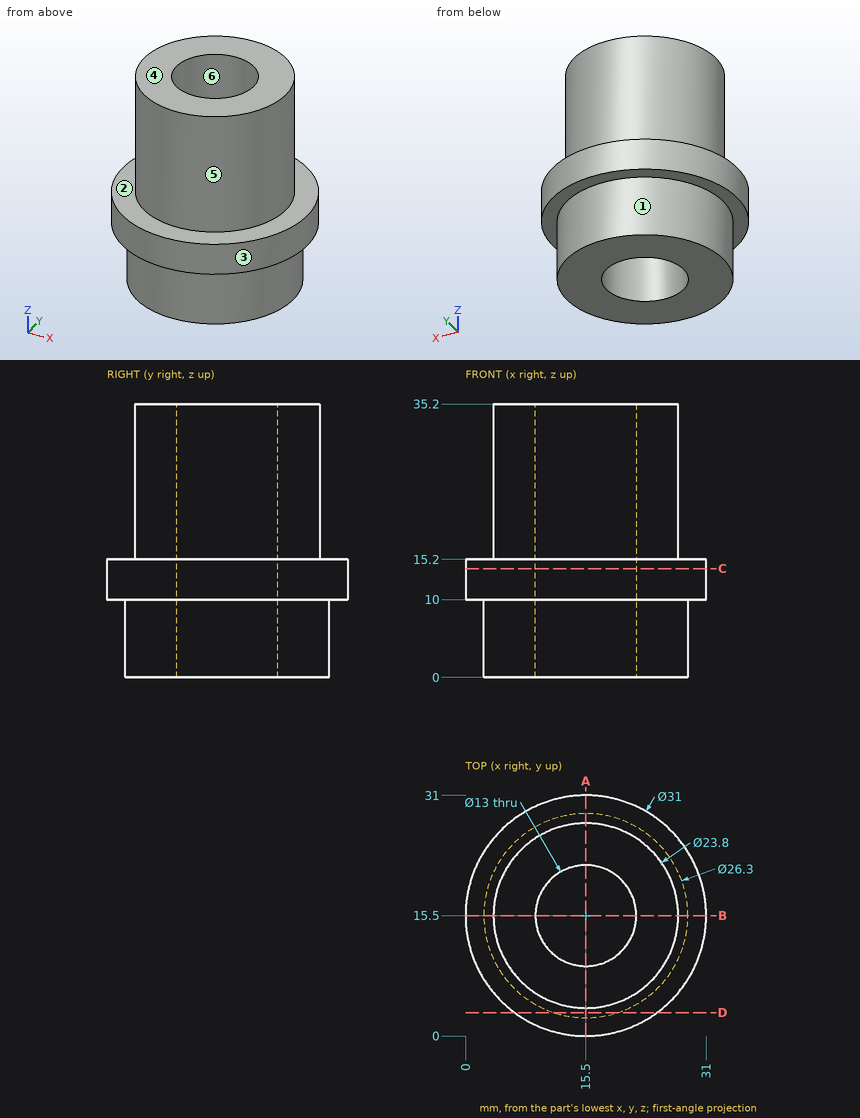
Verification items for this drawing (mm, ordinates from the low corner). A direction names the side the tool comes from. Round coordinates to 2 decimals unless told otherwise and drop trailing zeros. Write each loop counter-clockwise with the first axis right and the second up, starting at its lowest first coordinate (ties: lowest second). Pieces come first, ordered by that corner, then holes. Notation, with made-up numbers: M -27.5,50 L -6.5,50 A17 ccw -6.5,72 Z; hole C 72.25,-6 d9. An arc over 180 degrees is marked long. Write item = value, one per line. Start each with the question number.
1. Section check C-C, the plane z = 14. Record the cut outline in (x, y), then the cut area to 3 significant figures.
2. Section check A-A, the plane x = 15.5. Record the cut outline in (y, z).
3. Tool access check on the marked faces 1, 2 and 3. Record the directions out of +Z, -Z, +X, -X, +Y, -Y that give a thin tool (end or side, any length) a straight path to the whole face; none if there is none.
4. Section check D-D, the plane y = 3. Record the cut outline in (x, z).
5. Scan lines: line 1 (Y direction, x = 15.5, z = 13); line 2 (Y direction, x = 15.5, z = 21); line 3 (Z direction, x = 12.5, y = 2). Record each from-to range of solid material in increasing order. Write a range as [from, to].
6. Release check for a two-part mould opening along X. For the marked faces 4, 5 and 6 record: pulls with the +X half, pulls with the -X half, needs draft (parallel to the pull), parting line crosses it, or undercut.
7. Gauge pin test, flat ends, axial feed: pin 1 (5 mm diameter, centred on y = 14.5, z = 13.5, fed in from +X); pin 2 (4 mm diameter, centred on y = 13.5, z = 16, fed in from -X); pin 3 (1.5 mm diameter, centred on x = 14, z = 25.5, fed in from -Y). Record the tip position at first contact, or that the pin passes through.
Results found:
q1.outline = C 15.5,15.5 d31; hole C 15.5,15.5 d13
q1.area = 622 mm^2
q2.outline = M 0,10 L 2.35,10 L 2.35,0 L 9,0 L 9,35.2 L 3.6,35.2 L 3.6,15.2 L 0,15.2 Z; M 22,0 L 28.65,0 L 28.65,10 L 31,10 L 31,15.2 L 27.4,15.2 L 27.4,35.2 L 22,35.2 Z
q3.face_1 = -Z
q3.face_2 = +Z
q3.face_3 = +Z, -Z
q4.outline = M 6.33,10 L 11.42,10 L 11.42,0 L 19.58,0 L 19.58,10 L 24.67,10 L 24.67,15.2 L 6.33,15.2 Z
q5.line_1 = [0, 9], [22, 31]
q5.line_2 = [3.6, 9], [22, 27.4]
q5.line_3 = [10, 15.2]
q6.face_4 = needs draft
q6.face_5 = parting line crosses it
q6.face_6 = undercut
q7.pin_1 = 31
q7.pin_2 = 0
q7.pin_3 = 3.62
